The drawing under review shows one solid part. Ordinate dimensions are in mm from its lowest x, y, z. Coordinates: 2 decimals unless noted, no trailing zeros. Write each loop counter-clockwise with the first axis right and the second up, starting at its lowest first coordinate (ties: lowest second). Pieces come first, ordered by that corner, then holes.
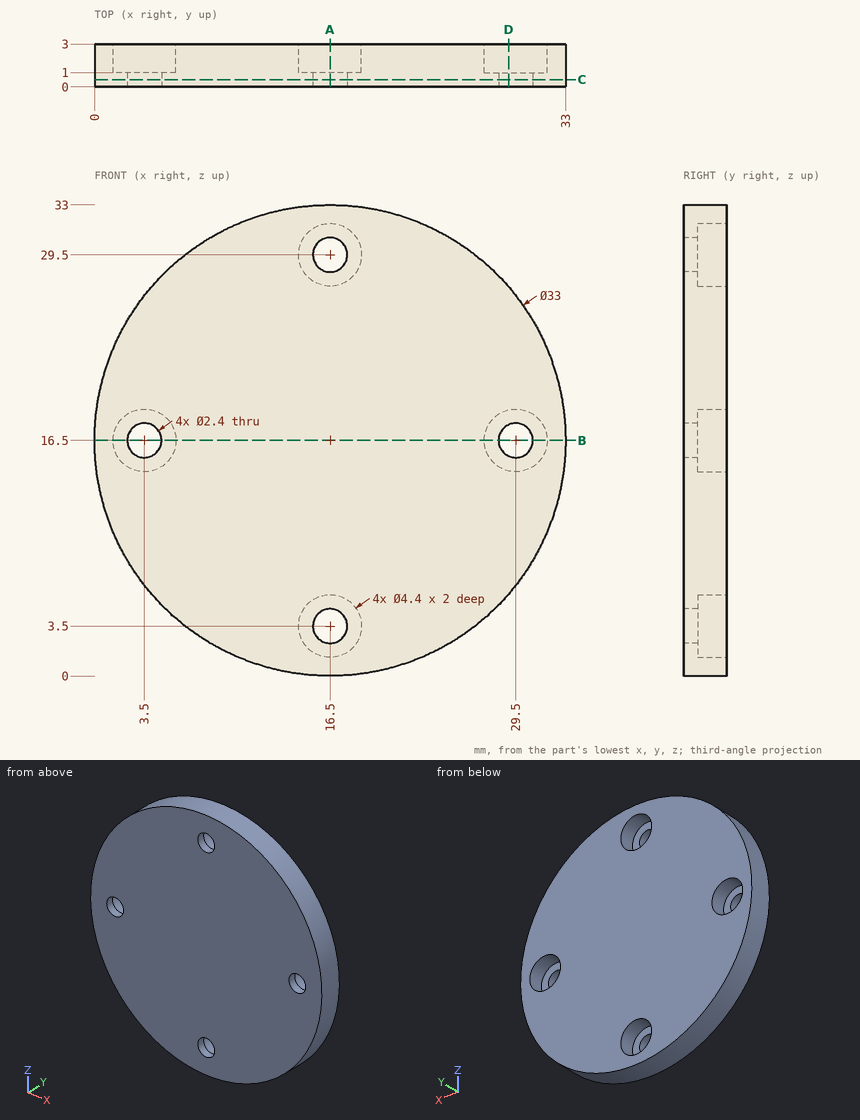
Q1. Add section D-D (x = 29). State the section outline as (y, z) points.
Ans:
outline: (0, 5.73) - (3, 5.73) - (3, 14.36) - (1, 14.36) - (1, 15.41) - (0, 15.41) - close; (0, 17.59) - (1, 17.59) - (1, 18.64) - (3, 18.64) - (3, 27.27) - (0, 27.27) - close
Q2. Add section B-B (z = 16.5). State the section outline as (x, y) points, then the cut area to 3 significant figures.
Ans:
outline: (0, 0) - (2.3, 0) - (2.3, 1) - (1.3, 1) - (1.3, 3) - (0, 3) - close; (4.7, 0) - (28.3, 0) - (28.3, 1) - (27.3, 1) - (27.3, 3) - (5.7, 3) - (5.7, 1) - (4.7, 1) - close; (30.7, 0) - (33, 0) - (33, 3) - (31.7, 3) - (31.7, 1) - (30.7, 1) - close
area: 76.6 mm2
Q3. Add section A-A (x = 16.5). State the section outline as (y, z) points, then the cut area to 3 significant figures.
Ans:
outline: (0, 0) - (3, 0) - (3, 1.3) - (1, 1.3) - (1, 2.3) - (0, 2.3) - close; (0, 4.7) - (1, 4.7) - (1, 5.7) - (3, 5.7) - (3, 27.3) - (1, 27.3) - (1, 28.3) - (0, 28.3) - close; (0, 30.7) - (1, 30.7) - (1, 31.7) - (3, 31.7) - (3, 33) - (0, 33) - close
area: 76.6 mm2
Q4. Clearance check with flat-ended pins moving along their axes: pin 1 Ø3 at (x, z) = (29.5, 16.5) entering from +Y; pin 2 Ø5.5 at (x, z) = (16.5, 3.5) entering from +Y; pin 3 Ø1 at (x, y) = (19, 2.5) entering from -Z; pin 4 Ø1 at (y, z) = (2.5, 7.5) entering from -X. State where each tip first meets the part, or that it passes through.
Ans:
pin 1: stops at y = 1
pin 2: stops at y = 3
pin 3: stops at z = 0.12
pin 4: stops at x = 2.36
Q5. For probe 1 along Z at (x, y) = (17, 2.2); probe 2 along Z at (x, y) = (29.5, 2.1), list the stretches that pass through material, from the lowest coordinate up.
Ans:
probe 1: z = 0.01 to 1.36, 5.64 to 27.36, 31.64 to 32.99
probe 2: z = 6.34 to 14.3, 18.7 to 26.66
Q6. Add section C-C (y = 0.5). State the section outline as (x, z) points.
Ans:
outline: circle Ø33 at (16.5, 16.5); hole circle Ø2.4 at (3.5, 16.5); hole circle Ø2.4 at (16.5, 3.5); hole circle Ø2.4 at (16.5, 29.5); hole circle Ø2.4 at (29.5, 16.5)
